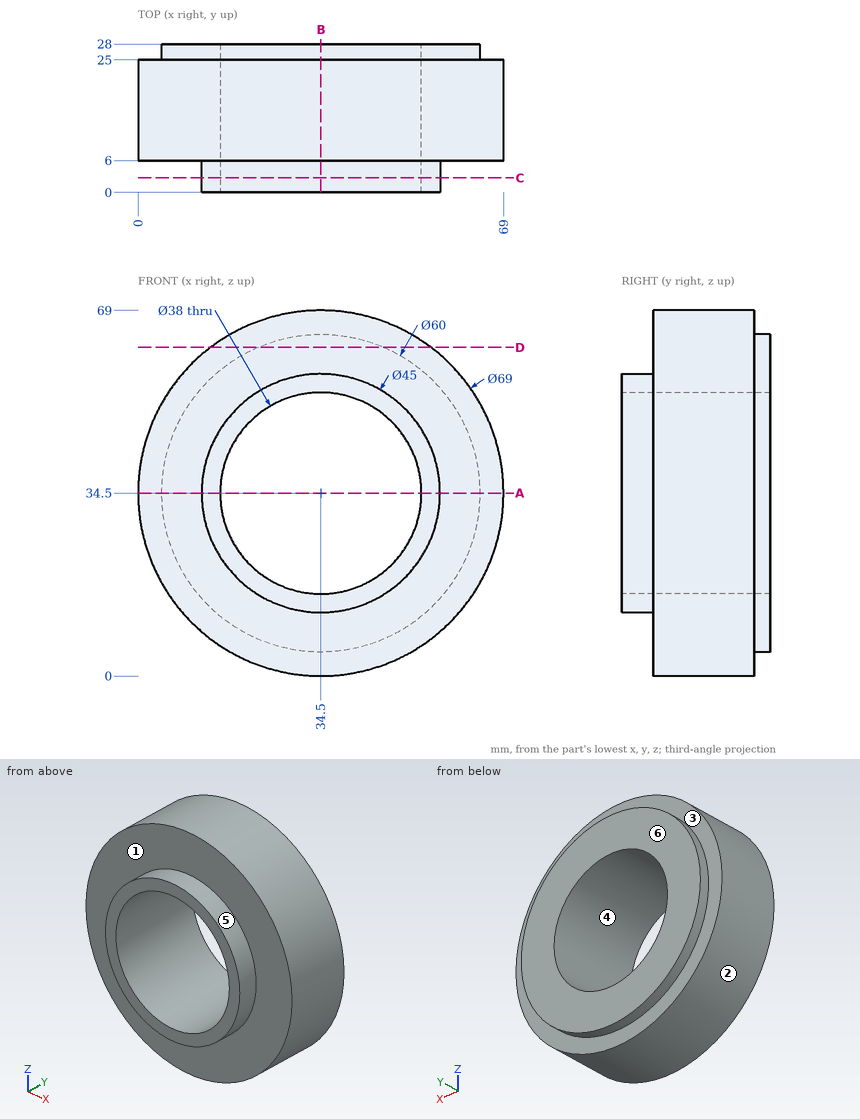
For this review, use the dimensioned drawing (mm, ordinates from the lowest corner) and the shaded views. A direction names the side the tool comes from. Round coordinates to 2 decimals unless told otherwise and drop trailing zeros. Order: outer loops, then holes, each group sorted by start corner. A loop starts at its lowest first (then second) coordinate and runs counter-clockwise, first axis right, second up. Notation, with made-up numbers: (63, 14.25) -> (97, 14.25) arc R28 ccw to (97, 48.25) -> close; hole circle Ø4 at (25, -34). An arc over 180 degrees is marked (long way). Write item = value, one per line. Start each with the question number.
Item 1: Mouldability with a two-part tool opening along Z and no side actions: class the marked faces 4, 5 and 6 as released by +Z, released by -Z, zero draft, split by the parting line, or undercut.
Item 2: Consider section D-D on z = 62. Write out the cut boundary in (x, y).
Item 3: For line 1 along Z through (x, y) = (34.5, 18.75); line 2 along Y through (x, z) = (13.5, 50); line 3 along Z through (x, y) = (48.5, 20), list the stretches that pass through material, from the lowest coordinate up.
Item 4: Clearance check with flat-ended pins moving along their axes: pin 1 Ø10 at (x, y) = (53.5, 23.5) entering from +Z; pin 2 Ø4 at (x, y) = (51.5, 13) entering from -Z; pin 3 Ø1.5 at (x, y) = (21.5, 14) entering from +Z. State where each tip first meets the part, or that it passes through.
Item 5: For the marked faces 1, 2 and 3, list the 3-axis set-ups (+Z, -Z, +X, -X, +Y, -Y) from which the entire face can be reached by the end or side of a thin tool; tool diameter is ignored.
Item 6: Consider section A-A on z = 34.5. Write out the cut boundary in (x, y), plus the area to 3 significant figures.
Item 7: Consider section B-B on x = 34.5. Write out the cut boundary in (y, z), plus the area to 3 significant figures.
Item 8: Consider section C-C on y = 2.75. Write out the cut boundary in (x, z), plus the area to 3 significant figures.
Conclusion:
q1.face_4 = undercut
q1.face_5 = split by the parting line
q1.face_6 = zero draft
q2.outline = (13.67, 6) -> (55.33, 6) -> (55.33, 25) -> (46.49, 25) -> (46.49, 28) -> (22.51, 28) -> (22.51, 25) -> (13.67, 25) -> close
q3.line_1 = 0 to 15.5, 53.5 to 69
q3.line_2 = 6 to 28
q3.line_3 = 2.97 to 21.65, 47.35 to 66.03
q4.pin_1 = 66.03
q4.pin_2 = 3.43
q4.pin_3 = 66.75
q5.face_1 = -Y
q5.face_2 = +Y, -Y
q5.face_3 = +Y
q6.outline = (0, 6) -> (12, 6) -> (12, 0) -> (15.5, 0) -> (15.5, 28) -> (4.5, 28) -> (4.5, 25) -> (0, 25) -> close; (53.5, 0) -> (57, 0) -> (57, 6) -> (69, 6) -> (69, 25) -> (64.5, 25) -> (64.5, 28) -> (53.5, 28) -> close
q6.area = 697 mm2
q7.outline = (0, 12) -> (6, 12) -> (6, 0) -> (25, 0) -> (25, 4.5) -> (28, 4.5) -> (28, 15.5) -> (0, 15.5) -> close; (0, 53.5) -> (28, 53.5) -> (28, 64.5) -> (25, 64.5) -> (25, 69) -> (6, 69) -> (6, 57) -> (0, 57) -> close
q7.area = 697 mm2
q8.outline = circle Ø45 at (34.5, 34.5); hole circle Ø38 at (34.5, 34.5)
q8.area = 456 mm2
